from build123d import *

# Parameters (mm, degrees)
SKETCH1_W           = 80
SKETCH1_H           = 73
BOSS_EXTRUDE1_DEPTH = 10
SKETCH3_R           = 3.25
CUT_EXTRUDE1_DEPTH  = 10
SKETCH4_W           = 80
SKETCH4_H           = 30
SKETCH4_R           = 11.5
BOSS_EXTRUDE2_DEPTH = 10
BOSS_EXTRUDE3_START = 6
SKETCH5_W           = 80
SKETCH5_H           = 29.5
SKETCH5_R           = 11.5
BOSS_EXTRUDE3_DEPTH = 6
SKETCH6_R           = 2.25
CUT_EXTRUDE2_DEPTH  = 28
SKETCH7_W           = 80
SKETCH7_H           = 30
CUT_EXTRUDE3_DEPTH  = 20
BOSS_EXTRUDE4_DEPTH = 10
SKETCH9_R           = 5.5
CUT_EXTRUDE4_DEPTH  = 6
FILLET1_R           = 3
SKETCH10_R          = 2.25
CUT_EXTRUDE5_DEPTH  = 16
CUT_EXTRUDE6_DEPTH  = 6


with BuildPart() as part:
    # Sketch1 → Boss-Extrude1 (new body)
    with BuildSketch(Plane(origin=(0, 0, 0), x_dir=(1, 0, 0), z_dir=(0, 1, 0))):
        with Locations((40, 36.5)):
            Rectangle(SKETCH1_W, SKETCH1_H)
    extrude(amount=BOSS_EXTRUDE1_DEPTH)

    # Sketch3 → Cut-Extrude1 (cut)
    with BuildSketch(Plane(origin=(0, 0, 0), x_dir=(-1, 0, 0), z_dir=(0, -1, 0))):
        with Locations(Location((-6.5, 6.5, 0), (0, 0, 90))):
            Circle(SKETCH3_R)
        with Locations(Location((-22.5, 6.5, 0), (0, 0, 90))):
            Circle(SKETCH3_R)
        with Locations(Location((-57.5, 6.5, 0), (0, 0, 90))):
            Circle(SKETCH3_R)
        with Locations(Location((-73.5, 6.5, 0), (0, 0, 90))):
            Circle(SKETCH3_R)
        with Locations(Location((-73.5, 66.5, 0), (0, 0, 270))):
            Circle(SKETCH3_R)
        with Locations(Location((-57.5, 66.5, 0), (0, 0, 270))):
            Circle(SKETCH3_R)
        with Locations(Location((-22.5, 66.5, 0), (0, 0, 270))):
            Circle(SKETCH3_R)
        with Locations(Location((-6.5, 66.5, 0), (0, 0, 270))):
            Circle(SKETCH3_R)
    extrude(amount=-CUT_EXTRUDE1_DEPTH, mode=Mode.SUBTRACT)

    # Sketch4 → Boss-Extrude2 (add)
    with BuildSketch(Plane(origin=(0, 10, 0), x_dir=(1, 0, 0), z_dir=(0, 1, 0))):
        with Locations((40, -15)):
            Rectangle(SKETCH4_W, SKETCH4_H)
        with Locations(Location((14, -14, 0), (0, 0, 270))):
            Circle(SKETCH4_R, mode=Mode.SUBTRACT)
        with Locations(Location((66, -14, 0), (0, 0, 270))):
            Circle(SKETCH4_R, mode=Mode.SUBTRACT)
    extrude(amount=-BOSS_EXTRUDE2_DEPTH)

    # Sketch5 → Boss-Extrude3 (add)
    with BuildSketch(Plane(origin=(0, 10, 0), x_dir=(1, 0, 0), z_dir=(0, 1, 0)).offset(BOSS_EXTRUDE3_START)):
        with Locations((40, -15.25)):
            Rectangle(SKETCH5_W, SKETCH5_H)
        with Locations(Location((14, -14, 0), (0, 0, 270))):
            Circle(SKETCH5_R, mode=Mode.SUBTRACT)
        with Locations(Location((66, -14, 0), (0, 0, 270))):
            Circle(SKETCH5_R, mode=Mode.SUBTRACT)
    extrude(amount=-BOSS_EXTRUDE3_DEPTH)

    # Sketch6 → Cut-Extrude2 (cut)
    with BuildSketch(Plane(origin=(0, 10, 0), x_dir=(1, 0, 0), z_dir=(0, 1, 0))):
        with Locations(Location((70.25, 29, 0), (0, 0, 270))):
            Circle(SKETCH6_R)
        with BuildLine():
            Line((37.5, 13.75), (37.5, 44.25))
            ThreePointArc((37.5, 44.25), (39.75, 46.5), (42, 44.25))
            Line((42, 44.25), (42, 13.75))
            ThreePointArc((42, 13.75), (39.75, 11.5), (37.5, 13.75))
        make_face()
    extrude(amount=-CUT_EXTRUDE2_DEPTH, mode=Mode.SUBTRACT)

    # Sketch7 → Cut-Extrude3 (cut)
    with BuildSketch(Plane(origin=(0, 16, 0), x_dir=(1, 0, 0), z_dir=(0, 1, 0))):
        with Locations((40, -15)):
            Rectangle(SKETCH7_W, SKETCH7_H)
    extrude(amount=-CUT_EXTRUDE3_DEPTH, mode=Mode.SUBTRACT)

    # Sketch8 → Boss-Extrude4 (add)
    with BuildSketch(Plane(origin=(0, 10, 0), x_dir=(1, 0, 0), z_dir=(0, 1, 0))):
        with BuildLine():
            Line((13, -4.602752641), (13, 0))
            Line((13, 0), (16, 0))
            Line((16, 0), (16, -4.602752641))
            ThreePointArc((16, -4.602752641), (14.5, -4.5), (13, -4.602752641))
        make_face()
        with BuildLine():
            Line((65, 0), (65, -4.602752641))
            ThreePointArc((65, -4.602752641), (66.5, -4.5), (68, -4.602752641))
            Line((68, -4.602752641), (68, 0))
            Line((68, 0), (65, 0))
        make_face()
    extrude(amount=-BOSS_EXTRUDE4_DEPTH)

    # Sketch9 → Cut-Extrude4 (cut)
    with BuildSketch(Plane(origin=(0, 10, 0), x_dir=(1, 0, 0), z_dir=(0, 1, 0))):
        with Locations(Location((57.5, 6.5, 0), (0, 0, 270))):
            Circle(SKETCH9_R)
        with BuildLine():
            Line((73.5, 0), (80, 0))
            Line((80, 0), (80, 6.5))
            ThreePointArc((80, 6.5), (68.903805922, 11.096194078), (73.5, 0))
        make_face()
    extrude(amount=-CUT_EXTRUDE4_DEPTH, mode=Mode.SUBTRACT)

    # Fillet1
    fillet1_edges = [part.edges().sort_by_distance(p)[0] for p in [
        (13, 5, 0),
        (16, 5, 0),
        (65, 5, 0),
        (68, 5, 0),
    ]]
    fillet(fillet1_edges, radius=FILLET1_R)

    # Sketch10 → Cut-Extrude5 (cut)
    with BuildSketch(Plane(origin=(0, 10, 0), x_dir=(1, 0, 0), z_dir=(0, 1, 0))):
        with Locations(Location((14.5, 16.5, 0), (0, 0, 270))):
            Circle(SKETCH10_R)
    extrude(amount=-CUT_EXTRUDE5_DEPTH, mode=Mode.SUBTRACT)

    # Sketch11 → Cut-Extrude6 (cut)
    with BuildSketch(Plane(origin=(0, 0, 0), x_dir=(-1, 0, 0), z_dir=(0, -1, 0))):
        Polygon((-10.458548116, 16.5), (-12.479274058, 20), (-16.520725942, 20), (-18.541451884, 16.5), (-16.520725942, 13), (-12.479274058, 13), align=None)
    extrude(amount=-CUT_EXTRUDE6_DEPTH, mode=Mode.SUBTRACT)


solid = part.part
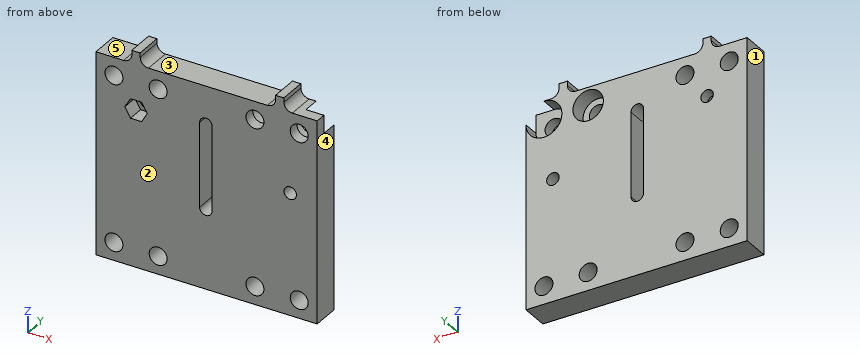
Verification items for the finished model (mm, model axes). Face numbers are marked on the shaded views. A direction names the side the tool comes from. Give positions to 0.01 mm unless a question says otherwise; leave off trailing zeros. Write each loop counter-clockwise with the first axis right and the second up, starting at its lowest first coordinate (ties: lowest second). Pieces come first, ordered by that corner, then holes. Notation, with made-up numbers: M 44,50 L 68,50 A24 cw 68,86 Z; hole C 21,8 d2. An arc over 180 degrees is marked long. Put each result on its own line as item: value. Start each with the question number.
1. Go/stop test with flat-tipped pins: pin 1 Ø4 at (x, z) = (22.5, -66.5) entering from +Y; pin 2 Ø5 at (y, z) = (2.5, -19.5) entering from -X; pin 3 Ø4.5 at (x, y) = (74.5, 7) entering from +Z; pin 4 Ø3.5 at (x, z) = (55.5, -8.5) entering from +Y. Record where each tip stops, or that it passes through.
2. Scan lines: line 1 along X through (y, z) = (7.75, -66.5); line 2 along X through (y, z) = (3.5, -39.5); line 3 along Z through (x, y) = (21, 9.25). Record each from-to range of solid material in increasing order. Write a range as [from, to].
3. Draft check along X on the marked faces 1, 2 and 3. Enter one of: +X half, -X half, draft (parallel to the pull), parting line (faces both ways), or undercut.
4. Section check D-D (x = 14.5). Record the cut outline in (y, z).
5. Section check C-C (z = -39). Record the cut outline in (x, y).
6. Section check B-B (x = 57.5). Record the cut outline in (y, z).
7. Set-up check for the marked faces 4 and 5: record each of +Z, -Z, +X, -X, +Y, -Y from which the full face is reachable in a straight line by a thin tool's end or side.
8. Section check A-A (y = 7). Give the number of separate pieces and of enclosed holes in the cut face, and give its area (3 significant figures).
Answer list:
1. pin 1: through
1. pin 2: x = 0
1. pin 3: z = 0
1. pin 4: y = 4
2. line 1: [0, 3.25], [9.75, 19.25], [25.75, 54.25], [60.75, 70.25], [76.75, 80]
2. line 2: [0, 37.5], [42, 80]
2. line 3: [-73, -69.38], [-63.62, -9.38], [-3.62, 0]
3. face 1: -X half
3. face 2: draft
3. face 3: undercut
4. outline: M 0,-73 L 10,-73 L 10,-18.75 L 6,-18.75 L 6,-20 L 0,-20 Z; M 0,-13 L 6,-13 L 6,-14.25 L 10,-14.25 L 10,4.5 L 0,4.5 Z
5. outline: M 0,0 L 37.5,0 L 37.5,10 L 0,10 Z; M 42,0 L 80,0 L 80,10 L 42,10 Z
6. outline: M 0,-73 L 10,-73 L 10,-69.75 L 0,-69.75 Z; M 0,-63.25 L 10,-63.25 L 10,-12 L 4,-12 L 4,-9.75 L 0,-9.75 Z; M 0,-3.25 L 4,-3.25 L 4,-1 L 10,-1 L 10,0 L 0,0 Z
7. face 4: +Z, -Z, +X, +Y, -Y
7. face 5: +Z, -X, +Y, -Y
8. separate pieces: 1
8. enclosed holes: 10
8. area: 5,250 mm2
